from build123d import *

# Parameters (mm, degrees)
SKETCH_2_W          = 41
SKETCH_2_H          = 9
EXTRUDE_1_DEPTH     = 30
SKETCH_3_R          = 1.6
CUT_EXTRUDE_1_DEPTH = 54.572380944
CUT_EXTRUDE_2_DEPTH = 3
CUT_EXTRUDE_3_DEPTH = 3
CUT_EXTRUDE_4_DEPTH = 3


with BuildPart() as part:
    # 草图2 → 凸台-拉伸1 (new body)
    with BuildSketch(Plane.XY):
        Polygon((0, 0), (-43, 0), (-43, 11), (0, 11), (0, 10), (0, 1), align=None)
        with Locations((-21.5, 5.5)):
            Rectangle(SKETCH_2_W, SKETCH_2_H, mode=Mode.SUBTRACT)
    extrude(amount=EXTRUDE_1_DEPTH)

    # 草图3 → 切除-拉伸1 (cut, through all)
    with BuildSketch(Plane(origin=(0, 11, 0), x_dir=(1, 0, 0), z_dir=(0, 1, 0))):
        with Locations(Location((-34, -7, 0), (0, 0, 270))):
            Circle(SKETCH_3_R)
        with Locations(Location((-34, -23, 0), (0, 0, 270))):
            Circle(SKETCH_3_R)
        with Locations(Location((-15.3, -23, 0), (0, 0, 270))):
            Circle(SKETCH_3_R)
        with Locations(Location((-12.5, -7, 0), (0, 0, 180))):
            Circle(SKETCH_3_R)
    extrude(amount=-CUT_EXTRUDE_1_DEPTH, mode=Mode.SUBTRACT)

    # 草图4 → 切除-拉伸2 (cut)
    with BuildSketch(Plane(origin=(0, 11, 0), x_dir=(1, 0, 0), z_dir=(0, 1, 0))):
        with BuildLine():
            Line((-19.3, 0), (-19.3, -3.2))
            ThreePointArc((-19.3, -3.2), (-23.3, -7.2), (-27.3, -3.2))
            Line((-27.3, -3.2), (-27.3, 0))
            Line((-27.3, 0), (-19.3, 0))
        make_face()
    extrude(amount=-CUT_EXTRUDE_2_DEPTH, mode=Mode.SUBTRACT)

    # 草图6 → 切除-拉伸3 (cut)
    with BuildSketch(Plane(origin=(0, 1, 0), x_dir=(1, 0, 0), z_dir=(0, 1, 0))):
        with BuildLine():
            Line((-28.3, -3.2), (-28.3, 0))
            Line((-28.3, 0), (-18.3, 0))
            Line((-18.3, 0), (-18.3, -3.2))
            ThreePointArc((-18.3, -3.2), (-23.3, -8.2), (-28.3, -3.2))
        make_face()
    extrude(amount=-CUT_EXTRUDE_3_DEPTH, mode=Mode.SUBTRACT)

    # 草图7 → 切除-拉伸4 (cut)
    with BuildSketch(Plane(origin=(0, 0, 0), x_dir=(0, 0, -1), z_dir=(1, 0, 0))):
        with BuildLine():
            Line((-7, 8.5), (0, 8.5))
            Line((0, 8.5), (0, 2.5))
            Line((0, 2.5), (-7, 2.5))
            ThreePointArc((-7, 2.5), (-10, 5.5), (-7, 8.5))
        make_face()
    extrude(amount=-CUT_EXTRUDE_4_DEPTH, mode=Mode.SUBTRACT)


solid = part.part
Part model, mm, in its own coordinate system. A direction names the side the tool comes from. Give positions to 0.01 mm unless a question says otherwise; leave off trailing zeros. Write each loop counter-clockwise with the first axis right and the second up, starting at its lowest first coordinate (ties: lowest second). Pieces come first, ordered by that corner, then holes.
1) Cut at B-B on y = 9.5. Write the cut outline in (x, z), then the cut area to 3 significant figures.
Resolved:
outline: (-43, 0) - (-42, 0) - (-42, 30) - (-43, 30) - close; (-1, 0) - (0, 0) - (0, 30) - (-1, 30) - close
area: 60.0 mm2
2) Cut at A-A on x = -15.3. Write the cut outline in (y, z).
Resolved:
outline: (0, 0) - (1, 0) - (1, 21.4) - (0, 21.4) - close; (0, 24.6) - (1, 24.6) - (1, 30) - (0, 30) - close; (10, 0) - (11, 0) - (11, 21.4) - (10, 21.4) - close; (10, 24.6) - (11, 24.6) - (11, 30) - (10, 30) - close
3) Cut at D-D on z = 23. Write the cut outline in (x, y), then the cut area to 3 significant figures.
Resolved:
outline: (-43, 0) - (-35.6, 0) - (-35.6, 1) - (-42, 1) - (-42, 10) - (-35.6, 10) - (-35.6, 11) - (-43, 11) - close; (-32.4, 0) - (-16.9, 0) - (-16.9, 1) - (-32.4, 1) - close; (-32.4, 10) - (-16.9, 10) - (-16.9, 11) - (-32.4, 11) - close; (-13.7, 0) - (0, 0) - (0, 11) - (-13.7, 11) - (-13.7, 10) - (-1, 10) - (-1, 1) - (-13.7, 1) - close
area: 91.2 mm2
4) Two-plate mould, pull along X, no slides. Class faces 5 (the face through (-27.3, 10.5, 1.6)), 6 (the face through (0, 5, 18)), 7 (the face through (-0.5, 2.5, 3.5)): released by +X, released by -X, zero draft, split by the parting line, or undercut.
Resolved:
face 5: undercut
face 6: released by +X
face 7: zero draft
5) Which spindle directions (+Z, -Z, +X, -X, +Y, -Y) get a long thin tool onto all of the face, cutting with end or side? Do faces 1 (the face through (-0.5, 5.4, 10)), 2 (the face through (-35.42, 10.51, 7.74)), 3 (the face through (-18.3, 0.5, 1.6)), 4 (the face through (-22, 1, 15)). Say none if no direction does.
Resolved:
face 1: -Z, +X
face 2: +Y, -Y
face 3: -Z, -Y
face 4: +Z, -Z
6) Probe L1, parallel to X at y = 0.35, z = 23; L2, parallel to X at y = 7.5, z = 23.5; L3, parallel to Y at x = -13, z = 11.5. List the from-to ranges inside material, lowest first.
Resolved:
L1: x = -43 to -35.6, -32.4 to -16.9, -13.7 to 0
L2: x = -43 to -42, -1 to 0
L3: y = 0 to 1, 10 to 11
7) Cut at C-C on x = -34. Write the cut outline in (y, z).
Resolved:
outline: (0, 0) - (1, 0) - (1, 5.4) - (0, 5.4) - close; (0, 8.6) - (1, 8.6) - (1, 21.4) - (0, 21.4) - close; (0, 24.6) - (1, 24.6) - (1, 30) - (0, 30) - close; (10, 0) - (11, 0) - (11, 5.4) - (10, 5.4) - close; (10, 8.6) - (11, 8.6) - (11, 21.4) - (10, 21.4) - close; (10, 24.6) - (11, 24.6) - (11, 30) - (10, 30) - close
8) Pin check, flat tip, straight feed: pin 1 (1 mm diameter, centred on x = -14.5, z = 22.5, fed in from +Y). Stop position of the tip, or through.
Resolved:
pin 1: passes through
